Read the model definition and answer for the solid it produces. Units are mm, in the model's axes. Give positions to 0.01 mm unless a question says otherwise; leave off trailing zeros. Write each loop counter-clockwise with the first axis right and the second up, starting at its lowest first coordinate (ties: lowest second). Pieces come first, ordered by that corner, then holes. Notation, with made-up numbers: (80, 60.25) -> (109, 60.25) arc R14 cw to (109, 69.25) -> close; hole circle Ø8 at (30, 80.25). An arc over 180 degrees is marked (long way). Use a Markdown table: item, result.
from build123d import *

# Parameters (mm, degrees)
F0_W     = 127
F0_H     = 127
F1_DEPTH = 63.5
F2_SIZE  = 25.4
F3_R     = 25.4
F4_DEPTH = 127.001
F5_R     = 6.35


with BuildPart() as f1:
    # F0 (on Front) → F1 (new body, symmetric)
    with BuildSketch(Plane.XZ):
        Rectangle(F0_W, F0_H)
    extrude(amount=F1_DEPTH, both=True)

    # F2
    f2_edges = [f1.edges().sort_by_distance(p)[0] for p in [
        (-63.5, 0, 63.5),
    ]]
    chamfer(f2_edges, length=F2_SIZE)

    # F3 (on face) → F4 (cut, through all)
    with BuildSketch(Plane(origin=(-63.5, 0, 0), x_dir=(0, -1, 0), z_dir=(-1, 0, 0))):
        Circle(F3_R)
    extrude(amount=-F4_DEPTH, mode=Mode.SUBTRACT)

    # F5
    f5_edges = [f1.edges().sort_by_distance(p)[0] for p in [
        (63.5, 63.5, 0),
        (63.5, 0, -63.5),
        (63.5, 0, 63.5),
        (63.5, -63.5, 0),
        (63.5, 25.4, 0),
    ]]
    fillet(f5_edges, radius=F5_R)


solid = f1.part
Item 1: A cutting plane is placed at B-B (z = 0). Give the vertices of the cut face in (x, y), then the cut area to 3 significant figures.
Return value:
| item | result |
|---|---|
| outline | (-63.5, -63.5) -> (57.15, -63.5) arc R6.35 ccw to (63.5, -57.15) -> (63.5, -31.75) arc R6.35 ccw to (57.15, -25.4) -> (-63.5, -25.4) -> close; (-63.5, 25.4) -> (57.15, 25.4) arc R6.35 ccw to (63.5, 31.75) -> (63.5, 57.15) arc R6.35 ccw to (57.15, 63.5) -> (-63.5, 63.5) -> close |
| area | 9,640 mm^2 |
Item 2: A cutting plane is placed at C-C (x = -41). Give the vertices of the cut face in (y, z), then the cut area to 3 significant figures.
Return value:
| item | result |
|---|---|
| outline | (-63.5, -63.5) -> (63.5, -63.5) -> (63.5, 60.6) -> (-63.5, 60.6) -> close; hole circle Ø50.8 at (0, 0) |
| area | 13,700 mm^2 |
Item 3: For a pull along Y with two mould halves and no side action, classify faces 1 (the face through (-4.02, 5.506, -24.796)), 2 (the face through (-4, -63.5, 1)), 3 (the face through (9, -1, 63.5)) as +Y half, -Y half, draft (parallel to the pull), parting line (faces both ways), or undercut.
Return value:
| item | result |
|---|---|
| face 1 | undercut |
| face 2 | -Y half |
| face 3 | draft |
Item 4: A cutting plane is placed at A-A (y = 0). Give the vertices of the cut face in (x, z).
Return value:
| item | result |
|---|---|
| outline | (-63.5, -63.5) -> (57.15, -63.5) arc R6.35 ccw to (63.5, -57.15) -> (63.5, -31.75) arc R6.35 ccw to (57.15, -25.4) -> (-63.5, -25.4) -> close; (-63.5, 25.4) -> (57.15, 25.4) arc R6.35 ccw to (63.5, 31.75) -> (63.5, 57.15) arc R6.35 ccw to (57.15, 63.5) -> (-38.1, 63.5) -> (-63.5, 38.1) -> close |
Item 5: Straight lines are drawn through the part: line 1 along Z through (x, y) = (-31, 0); line 2 along Y through (x, z) = (17, -4.5); line 3 along Z through (x, y) = (1.5, -16). For each, find the intervals that lie inside material, in ascending order. Write a range as [from, to].
Return value:
| item | result |
|---|---|
| line 1 | [-63.5, -25.4], [25.4, 63.5] |
| line 2 | [-63.5, -25], [25, 63.5] |
| line 3 | [-63.5, -19.73], [19.73, 63.5] |
Item 6: A cutting plane is placed at D-D (x = 45.5). Give the vertices of the cut face in (y, z), then the cut area to 3 significant figures.
Return value:
| item | result |
|---|---|
| outline | (-63.5, -63.5) -> (63.5, -63.5) -> (63.5, 63.5) -> (-63.5, 63.5) -> close; hole circle Ø50.8 at (0, 0) |
| area | 14,100 mm^2 |
